Part model, mm, in its own coordinate system. Round coordinates to 2 decimals unless told otherwise and drop trailing zeros. Loops run counter-clockwise (first coordinate to the right, second up) from the corner with the lowest first, then second, coordinate; pieces in that order, holes last. Notation, with made-up numbers: (17.25, -30) -> (29.25, -30) arc R13 ccw to (29.25, -24) -> close; hole circle Ø5 at (80, -27). An arc over 180 degrees is marked (long way). Use a Markdown table: item, result. Add a question column.
Item 1: Flat gauge pin, fed straight in: pin 1 (21 mm diameter, centred on x = -131.31, y = -1.42, fed in from +Z). Where does the tip first touch, or does it go through?
Item 2: Cut at B-B, the plane y = -38. List the corners of the cut face in (x, z).
Item 3: Two-plate mould, pull along Y, no slides. Class faces 1 (the face through (2.1, -39.97, 1.48)), 2 (the face through (94.687, -34.952, 1.521)), 3 (the face through (66.345, 43.176, 1.479)): pulls with the +Y half, pulls with the -Y half, needs draft (parallel to the pull), parting line crosses it, or undercut.
Item 4: Cut at A-A, the plane x = 55. List the corners of the cut face in (y, z), plus the area to 3 significant figures.
Item 5: Probe line 1 (Y direction, x = 94, z = 1.9); line 2 (Y direction, x = 107.5, z = 2.85); line 3 (X direction, y = 25, z = 0.8). List the from-to ranges inside material, lowest first. Write a range as [from, to].
Item 6: Cut at D-D, the plane z = 1.4. State how many separate pieces and enclosed holes the cut face has, plus the area to 3 significant figures.
Item 7: Cut at C-C, the plane x = 120. List the corners of the cut face in (y, z), plus the area to 3 significant figures.
```python
from build123d import *

# Parameters (mm, degrees)
BOSS_EXTRUDE1_DEPTH = 3
SKETCH2_R           = 8.006187357
SKETCH2_R_2         = 9.735262488
SKETCH2_R_3         = 13.182196279
SKETCH2_R_4         = 13.691397608
SKETCH2_R_5         = 19.450771096
SKETCH2_R_6         = 18.813943393
SKETCH2_R_7         = 18.770594662
SKETCH2_R_8         = 13.863766026
SKETCH2_R_9         = 10.613691542
CUT_EXTRUDE1_DEPTH  = 3


with BuildPart() as part:
    # Sketch1 → Boss-Extrude1 (new body)
    with BuildSketch(Plane.XY):
        Polygon((150, 56.603970605), (150, -63.396029395), (-150, -15.880697298), (-150, 9.119302702), (-15, 9.119302702), (-15, 30.119302702), align=None)
    extrude(amount=BOSS_EXTRUDE1_DEPTH)

    # Sketch2 → Cut-Extrude1 (cut)
    with BuildSketch(Plane.XY.offset(3)):
        with Locations((-131.306408306, -1.418891545)):
            Circle(SKETCH2_R)
        with Locations((-97.648790291, -4.870954931)):
            Circle(SKETCH2_R_2)
        with Locations((-60.754862852, -7.891510394)):
            Circle(SKETCH2_R_3)
        with Locations((-14.583515063, -9.425078902)):
            Circle(SKETCH2_R_4)
        with Locations((110.12227476, -23.116476509)):
            Circle(SKETCH2_R_5)
        with Locations((110.12227476, 26.629123467)):
            Circle(SKETCH2_R_6)
        with Locations((67.618744319, 5.290685885)):
            Circle(SKETCH2_R_7)
        with Locations((31.803586688, -19.757978284)):
            Circle(SKETCH2_R_8)
        with Locations((14.974777681, 17.567457079)):
            Circle(SKETCH2_R_9)
    extrude(amount=-CUT_EXTRUDE1_DEPTH, mode=Mode.SUBTRACT)


solid = part.part
```
A:
| question | item | result |
|---|---|---|
| 1 | pin 1 | stops at z = 3 |
| 2 | outline | (-10.34, 0) -> (97.6, 0) -> (97.6, 3) -> (-10.34, 3) -> close; (122.64, 0) -> (150, 0) -> (150, 3) -> (122.64, 3) -> close |
| 3 | face 1 | pulls with the -Y half |
| 3 | face 2 | undercut |
| 3 | face 3 | pulls with the +Y half |
| 4 | outline | (-48.35, 0) -> (-8.61, 0) -> (-8.61, 3) -> (-48.35, 3) -> close; (19.19, 0) -> (41.36, 0) -> (41.36, 3) -> (19.19, 3) -> close |
| 4 | area | 186 mm^2 |
| 5 | line 1 | y = [-54.53, -34], [-12.24, 16.93], [36.33, 47.62] |
| 5 | line 2 | y = [-56.66, -42.39], [-3.84, 8], [45.26, 49.78] |
| 5 | line 3 | x = [-15, 7.4], [22.55, 91.38], [128.87, 150] |
| 6 | separate pieces | 1 |
| 6 | enclosed holes | 9 |
| 6 | area | 14,300 mm^2 |
| 7 | outline | (-58.64, 0) -> (-39.87, 0) -> (-39.87, 3) -> (-58.64, 3) -> close; (-6.36, 0) -> (10.62, 0) -> (10.62, 3) -> (-6.36, 3) -> close; (42.64, 0) -> (51.79, 0) -> (51.79, 3) -> (42.64, 3) -> close |
| 7 | area | 135 mm^2 |
